from build123d import *

# Parameters (mm, degrees)
SKETCH1_R           = 0.75
SKETCH1_R_2         = 0.5
BOSS_EXTRUDE1_DEPTH = 2


with BuildPart() as part:
    # Sketch1 → Boss-Extrude1 (new body)
    with BuildSketch(Plane.XY):
        with BuildLine():
            Line((12.2, 4), (16.2, 4))
            Line((16.2, 4), (16.2, 2))
            ThreePointArc((16.2, 2), (15.614213562, 0.585786438), (14.2, 0))
            Line((14.2, 0), (2, 0))
            ThreePointArc((2, 0), (0.585786438, 0.585786438), (0, 2))
            Line((0, 2), (0, 4))
            Line((0, 4), (4, 4))
            Line((4, 4), (4, 6))
            Line((4, 6), (0, 6))
            Line((0, 6), (0, 15))
            Line((0, 15), (4, 15))
            Line((4, 15), (4, 17))
            Line((4, 17), (0, 17))
            Line((0, 17), (0, 20.23))
            ThreePointArc((0, 20.23), (1.464466094, 23.765533906), (5, 25.23))
            Line((5, 25.23), (11.2, 25.23))
            ThreePointArc((11.2, 25.23), (14.735533906, 23.765533906), (16.2, 20.23))
            Line((16.2, 20.23), (16.2, 17))
            Line((16.2, 17), (12.2, 17))
            Line((12.2, 17), (12.2, 15))
            Line((12.2, 15), (16.2, 15))
            Line((16.2, 15), (16.2, 6))
            Line((16.2, 6), (12.2, 6))
            Line((12.2, 6), (12.2, 4))
        make_face()
        with Locations((13.45, 2)):
            Circle(SKETCH1_R, mode=Mode.SUBTRACT)
        with Locations((13.2, 22.23)):
            Circle(SKETCH1_R_2, mode=Mode.SUBTRACT)
        with Locations((10.2, 8.5)):
            Circle(SKETCH1_R, mode=Mode.SUBTRACT)
        with Locations((13.45, 19)):
            Circle(SKETCH1_R, mode=Mode.SUBTRACT)
        with Locations((10.2, 12.5)):
            Circle(SKETCH1_R, mode=Mode.SUBTRACT)
        with Locations((6, 12.5)):
            Circle(SKETCH1_R, mode=Mode.SUBTRACT)
        with Locations((2.75, 19)):
            Circle(SKETCH1_R, mode=Mode.SUBTRACT)
        with Locations((6, 8.5)):
            Circle(SKETCH1_R, mode=Mode.SUBTRACT)
        with Locations((3, 22.23)):
            Circle(SKETCH1_R_2, mode=Mode.SUBTRACT)
        with Locations((2.75, 2)):
            Circle(SKETCH1_R, mode=Mode.SUBTRACT)
    extrude(amount=BOSS_EXTRUDE1_DEPTH)


solid = part.part
The listing builds one solid part. Answer for the finished solid, in the listing's coordinates (mm). A direction names the side the tool comes from. Coordinates: 2 decimals unless noted, no trailing zeros. Write each loop counter-clockwise with the first axis right and the second up, starting at its lowest first coordinate (ties: lowest second). Pieces come first, ordered by that corner, then holes. Notation, with made-up numbers: (-17.5, 32) - (23.5, 32) arc R23 cw to (23.5, 56) - close; hole circle Ø8 at (-3.75, 89.25). An arc over 180 degrees is marked (long way). Answer as CSV lines item,"result".
1. Determine the mould class of faces 4 (the flat face through (16.2, 11, 1)), 5 (the cylindrical face through (14.7, 23.8, 1)), 6 (the flat face through (4, 5, 1)) for opening direction Y: +Y half, -Y half, draft (parallel to the pull), parting line (faces both ways), or undercut.
Computed values:
face 4,"draft"
face 5,"+Y half"
face 6,"undercut"
2. Straight lines are drawn through the part: line 1 (Y direction, x = 10.2, z = 0.9); line 2 (Y direction, x = 2.75, z = 0.8); line 3 (Y direction, x = 13.2, z = 0.45). For each, find the intervals that lie inside material, in ascending order. Write a range as [from, to].
Computed values:
line 1,"y = [0, 7.75], [9.25, 11.75], [13.25, 25.23]"
line 2,"y = [0, 1.25], [2.75, 4], [6, 15], [17, 18.25], [19.75, 21.8], [22.66, 24.7]"
line 3,"y = [0, 1.29], [2.71, 4], [6, 15], [17, 18.29], [19.71, 21.73], [22.73, 24.81]"
3. Find section A-A (x = 10.2). Give the vertices of the cut face in (y, z), plus the area to 3 significant figures.
Computed values:
outline,"(0, 0) - (7.75, 0) - (7.75, 2) - (0, 2) - close; (9.25, 0) - (11.75, 0) - (11.75, 2) - (9.25, 2) - close; (13.25, 0) - (25.23, 0) - (25.23, 2) - (13.25, 2) - close"
area,"44.5 mm²"
4. Find section B-B (y = 19). Give the vertices of the cut face in (x, z).
Computed values:
outline,"(0, 0) - (2, 0) - (2, 2) - (0, 2) - close; (3.5, 0) - (12.7, 0) - (12.7, 2) - (3.5, 2) - close; (14.2, 0) - (16.2, 0) - (16.2, 2) - (14.2, 2) - close"
5. Find section C-C (z = 1.05). Give the number of separate pieces and of enclosed holes in the cut face, plus the area to 3 significant figures.
Computed values:
separate pieces,"1"
enclosed holes,"10"
area,"349 mm²"
6. Find section D-D (x = 13.2). Give the vertices of the cut face in (y, z), plus the area to 3 significant figures.
Computed values:
outline,"(0, 0) - (1.29, 0) - (1.29, 2) - (0, 2) - close; (2.71, 0) - (4, 0) - (4, 2) - (2.71, 2) - close; (6, 0) - (15, 0) - (15, 2) - (6, 2) - close; (17, 0) - (18.29, 0) - (18.29, 2) - (17, 2) - close; (19.71, 0) - (21.73, 0) - (21.73, 2) - (19.71, 2) - close; (22.73, 0) - (24.81, 0) - (24.81, 2) - (22.73, 2) - close"
area,"34.0 mm²"
7. A tool of negligible diameter and unlimited length cuts with its end or side. For faces 1 (the flat face through (12.2, 5, 1)), 2 (the flat face through (0, 3, 1)), 3 (the flat face through (2, 17, 1)), from which of +Z, -Z, +X, -X, +Y, -Y can it reach the whole face along a straight path? Write none if from no direction.
Computed values:
face 1,"+Z, -Z, +X"
face 2,"+Z, -Z, -X, +Y, -Y"
face 3,"+Z, -Z, -X"
8. Given P1, Ø1, axis at x = 14.5, z = 0.5, coming from the +Y side; P2, Ø0.6, axis at y = 15.5, z = 1, coming from the +X side; P3, Ø1, axis at x = 3, z = 1.5, coming from the +Y side, each flat-ended and moving along its own axis, determine where each tip first touches the part or whether it passes through.
Computed values:
P1,"stops at y = 24.37"
P2,"stops at x = 12.2"
P3,"stops at y = 25"
